```python
from build123d import *

# Parameters (mm, degrees)
FILLET1_R   = 0.2
FILLET2_R   = 0.4
HEX_2_DEPTH = 2


with BuildPart() as part:
    # BodySke → Base-Revolve (revolve)
    with BuildSketch(Plane.XY, mode=Mode.PRIVATE) as base_revolve_sk:
        Polygon((0, 0), (0, 3.5), (4, 3.5), (4, 2), (11.61, 2), (12, 1.61), (12, 0), align=None)
    revolve(base_revolve_sk.sketch.rotate(Axis((-31.75, 0, 0), (1, 0, 0)), 90), axis=Axis((-31.75, 0, 0), (1, 0, 0)))

    # Fillet1
    fillet1_edges = [part.edges().sort_by_distance(p)[0] for p in [
        (4, 0, -2),
    ]]
    fillet(fillet1_edges, radius=FILLET1_R)

    # Fillet2
    fillet2_edges = [part.edges().sort_by_distance(p)[0] for p in [
        (0, 0, -3.5),
    ]]
    fillet(fillet2_edges, radius=FILLET2_R)

    # Sketch2 → Hex-PreBroach (revolve, cut)
    with BuildSketch(Plane.XY, mode=Mode.PRIVATE) as hex_prebroach_sk:
        Polygon((0, 1.51), (2, 1.51), (2.871798906, 0), (0, 0), align=None)
    revolve(hex_prebroach_sk.sketch.rotate(Axis((0, 0, 0), (1, 0, 0)), 90), axis=Axis((0, 0, 0), (1, 0, 0)), mode=Mode.SUBTRACT)

    # Sketch3 → Hex 2 (cut)
    with BuildSketch(Plane(origin=(0, 0, 0), x_dir=(0, 0.500000000000001, 0.866025403784438), z_dir=(-1, 0, 0))):
        Polygon((0.871798906, 1.51), (-0.871798906, 1.51), (-1.743597813, 0), (-0.871798906, -1.51), (0.871798906, -1.51), (1.743597813, 0), align=None)
    extrude(amount=-HEX_2_DEPTH, mode=Mode.SUBTRACT)


solid = part.part
```
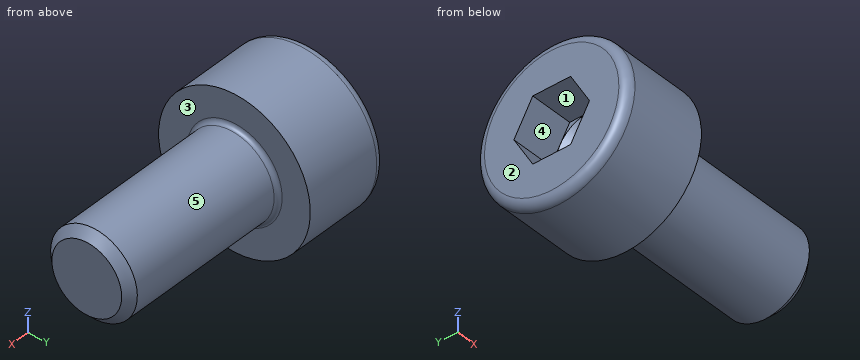
For this review, take the finished solid that the model builds, in its own axes (mm). Face numbers are marked on the shaded views. A direction names the side the tool comes from. Give positions to 0.01 mm unless a question says otherwise; leave off trailing zeros. Write each loop counter-clockwise with the first axis right and the second up, starting at its lowest first coordinate (ties: lowest second). Pieces come first, ordered by that corner, then holes.
Item 1: Machinability: for the marked faces 1 and 2, which of the approach directions +Z, -Z, +X, -X, +Y, -Y give a long, thin tool a straight path to every point of the face, cutting with its end or side? Answer none if there is none.
Item 2: Wall thickness on probe 1 along X at (y, z) = (2.5, 0); probe 2 along Z at (x, y) = (1.25, -0.75); probe 3 along Z at (x, y) = (1.75, 1.25): over which ranges is each line inside the solid? List them lowest first.
Item 3: Insertion check: P1, Ø1.5, axis at y = -2, z = 2.5, coming from the +X side; P2, Ø1.5, axis at x = 6, z = -2, coming from the +Y side; P3, Ø1.5, axis at x = 8.5, y = -1.5, coming from the +Z side. Each pin has a flat end and moves straight along its axis. Give the tip position at first contact, or say it passes through.
Item 4: Take a section at A-A (x = 3). Give the boundary of the cut face in (y, z), and give its area (3 significant figures).
Item 5: The part is to be moulded in two halves that separate along Z. For the marked faces 3, 4 and 5, say which applies: +Z half, -Z half, draft (parallel to the pull), parting line (faces both ways), or undercut.
Item 6: Take a section at B-B (x = 9.25). Give the boundary of the cut face in (y, z).
Established:
1. face 1: -X
1. face 2: +Z, -Z, -X, +Y, -Y
2. probe 1: x = 0 to 4
2. probe 2: z = -3.42 to -1.51, 1.51 to 3.42
2. probe 3: z = -3.27 to -0.85, 0.85 to 3.27
3. P1: stops at x = 4
3. P2: stops at y = 1.56
3. P3: stops at z = 1.85
4. outline: circle Ø7 at (0, 0)
4. area: 38.5 mm2
5. face 3: draft
5. face 4: undercut
5. face 5: parting line
6. outline: circle Ø4 at (0, 0)
